Check sheet for the drawn part. Datum: minimum x, y, z corner. Units: mm. A direction names the side the tool comes from. Coordinates: 2 decimals unless noted, no trailing zeros. Order: outer loops, then holes, each group sorted by start corner. A loop starts at its lowest first (then second) coordinate and runs counter-clockwise, first axis right, second up.
Q1. Cross-section at D-D, the plane z = 1.7. Record the boundary of the cut face in (x, y), and give its area (3 significant figures).
Q2. Cross-section at A-A, the plane y = 12.7. Record the boundary of the cut face in (x, z) (3 decimals).
Q3. Cross-section at C-C, the plane z = 3.6. Record the boundary of the cut face in (x, y).
Q4. Thickness scan on line 1 (Z direction, x = 23.25, y = 18.25); line 2 (Y direction, x = 13, z = 1.35); line 3 (Z direction, x = 16.75, y = 14). Record the ranges inside material, lowest first.
Q5. Set-up check for the marked faces 1 and 2: record each of +Z, -Z, +X, -X, +Y, -Y from which the full face is reachable in a straight line by a thin tool's end or side.
Q6. Depth check by flat-ended pin: P1, Ø2, axis at x = 4, z = 1, coming from the -Y side; P2, Ø5, axis at x = 22, y = 22.5, coming from the +Z side; P3, Ø1.5, axis at y = 19, z = 1, coming from the +X side. Enter the tip coordinate at first touch or a pass-through.
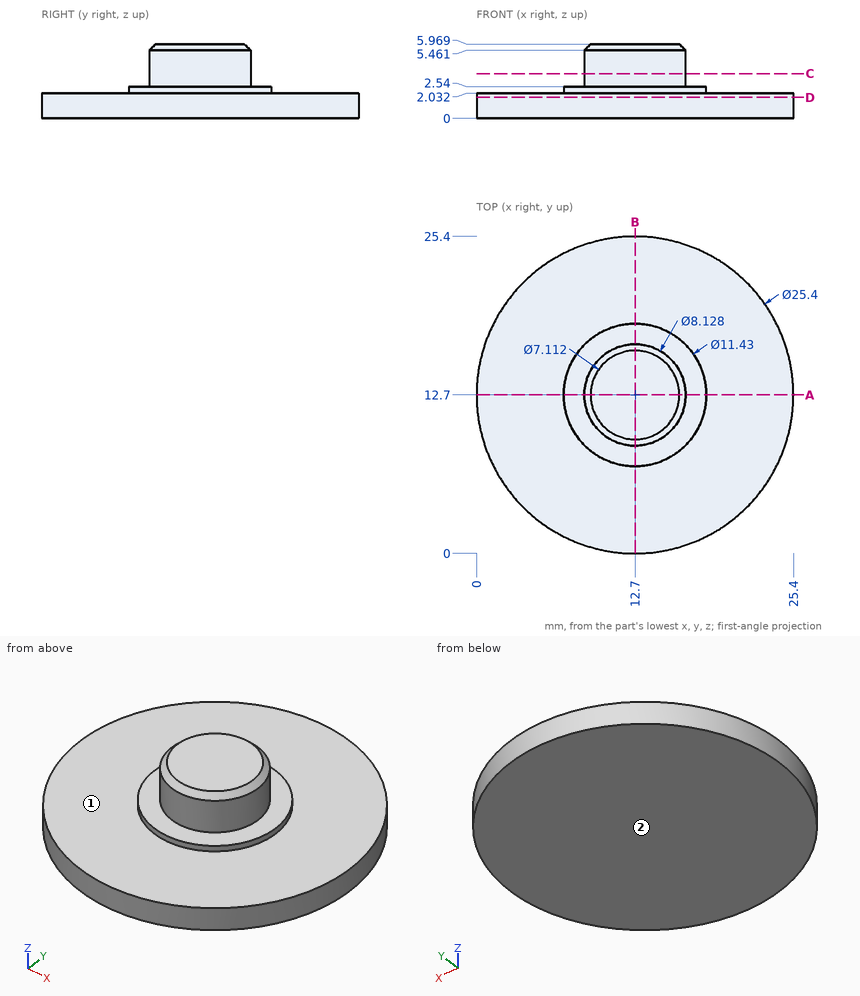
Check values:
1. outline: circle Ø25.4 at (12.7, 12.7)
1. area: 507 mm2
2. outline: (0, 0) - (25.4, 0) - (25.4, 2.032) - (18.415, 2.032) - (18.415, 2.54) - (16.764, 2.54) - (16.764, 5.461) - (16.256, 5.969) - (9.144, 5.969) - (8.636, 5.461) - (8.636, 2.54) - (6.985, 2.54) - (6.985, 2.032) - (0, 2.032) - close
3. outline: circle Ø8.13 at (12.7, 12.7)
4. line 1: z = 0 to 2.03
4. line 2: y = 0 to 25.4
4. line 3: z = 0 to 2.54
5. face 1: +Z
5. face 2: -Z, +X, -X, +Y, -Y
6. P1: stops at y = 2.6
6. P2: stops at z = 2.03
6. P3: stops at x = 24.12
